Model file for the job. Use its own axes, mm. A direction names the side the tool comes from. Coordinates: 2 decimals unless noted, no trailing zeros. Loops run counter-clockwise (first coordinate to the right, second up) from the corner with the lowest first, then second, coordinate; pieces in that order, holes last. Notation, with made-up numbers: (33.25, -38.75) -> (44.25, -38.75) arc R30 cw to (44.25, -6.75) -> close; hole circle Ø2 at (23.25, -18). An arc over 180 degrees is marked (long way). Use one line per item in the form item = value.
```python
from build123d import *

# Parameters (mm, degrees)
CROQUIS1_R              = 29.72
CROQUIS1_R_2            = 25.4
SALIENTE_EXTRUIR1_DEPTH = 100
CORTAR_EXTRUIR2_DEPTH   = 109.473760883
CROQUIS4_W              = 16
CROQUIS4_H              = 17
CORTAR_EXTRUIR3_DEPTH   = 109.47376103


with BuildPart() as part:
    # Croquis1 → Saliente-Extruir1 (new body)
    with BuildSketch(Plane.XY):
        Circle(CROQUIS1_R)
        Circle(CROQUIS1_R_2, mode=Mode.SUBTRACT)
    extrude(amount=SALIENTE_EXTRUIR1_DEPTH)

    # Croquis3 → Cortar-Extruir2 (cut, through all)
    with BuildSketch(Plane(origin=(0, 0, 0), x_dir=(0, 0, -1), z_dir=(1, 0, 0))):
        with BuildLine():
            Line((0, 21), (-21, 21))
            ThreePointArc((-21, 21), (-42, 0), (-21, -21))
            Line((-21, -21), (0, -21))
            Line((0, -21), (0, 21))
        make_face()
    extrude(amount=-CORTAR_EXTRUIR2_DEPTH, mode=Mode.SUBTRACT)

    # Croquis4 → Cortar-Extruir3 (cut, through all)
    with BuildSketch(Plane(origin=(0, 0, 0), x_dir=(0, 0, -1), z_dir=(1, 0, 0))):
        with Locations((-8, 0)):
            Rectangle(CROQUIS4_W, CROQUIS4_H)
    extrude(amount=CORTAR_EXTRUIR3_DEPTH, mode=Mode.SUBTRACT)


solid = part.part
```
Q1. Band-saw the part on C-C, the plane z = 80.5. Write the cut outline in (x, y), and give its area (3 significant figures).
Result:
outline = circle Ø59.44 at (0, 0); hole circle Ø50.8 at (0, 0)
area = 748 mm2
Q2. Which spindle directions (+Z, -Z, +X, -X, +Y, -Y) get a long thin tool onto all of the face, cutting with end or side? Do faces 1 (the face through (27, 0, 16)), 2 (the face through (22, 13, 100)), 3 (the face through (-18, -21, 11)). Say none if no direction does.
Result:
face_1 = -Z, +X, -X
face_2 = +Z, +X, -X, +Y, -Y
face_3 = -Z, -X
Q3. Pin check, flat tips, straight feed: pin 1 Ø2.5 at (x, z) = (25.5, 6) entering from -Y; pin 2 Ø4 at (y, z) = (23.5, 55.5) entering from +X; pin 3 Ø4 at (y, z) = (4.5, 51.5) entering from +X. Stop position of each tip, or through.
Result:
pin_1 = -17.18
pin_2 = 20.52
pin_3 = 29.61
Q4. Band-saw the part on D-D, the plane z = 22.5. Write the cut outline in (x, y).
Result:
outline = (-21.08, -20.95) arc R29.72 ccw (long way) to (-21.08, 20.95) -> (-14.37, 20.95) arc R25.4 cw (long way) to (-14.37, -20.95) -> close
Q5. Mould opens along X. For faces 4 (the face through (28.348, 8.927, 49.3)), 5 (the face through (23.463, -9.728, 60.411)), 6 (the face through (26, 8.5, 8)) say: released by +X, released by -X, zero draft, split by the parting line, or undercut.
Result:
face_4 = split by the parting line
face_5 = undercut
face_6 = zero draft
Q6. Band-saw the part on B-B, the plane y = 0. Write the cut outline in (x, z).
Result:
outline = (-29.72, 42) -> (-25.4, 42) -> (-25.4, 100) -> (-29.72, 100) -> close; (25.4, 16) -> (29.72, 16) -> (29.72, 100) -> (25.4, 100) -> close
Q7. Band-saw the part on A-A, the plane x = 0. Write the cut outline in (y, z).
Result:
outline = (-29.72, 0) -> (-25.4, 0) -> (-25.4, 100) -> (-29.72, 100) -> close; (25.4, 0) -> (29.72, 0) -> (29.72, 100) -> (25.4, 100) -> close
Q8. Wall check: line 1 along Y through (x, z) = (0, 74.5); line 2 along Y through (x, z) = (8, 86). Give the ranges that are in metal, low to high.
Result:
line_1 = -29.72 to -25.4, 25.4 to 29.72
line_2 = -28.62 to -24.11, 24.11 to 28.62
